Can you work these out from the model? Positions are in its coordinate system, mm. A direction names the side the tool comes from. Give positions to 0.01 mm unless a question says otherwise; leave off trailing zeros. Write each loop counter-clockwise with the first axis right and the second up, starting at its lowest first coordinate (ties: lowest second). Pieces come first, ordered by that corner, then holes. Notation, with made-up numbers: M 11,5.25 L 34,5.25 A17 ccw 34,36.25 Z; hole C -7,6.5 d10. An arc over 180 degrees is marked long. Write each question's results on one line, items separated by ' | '.
from build123d import *

# Parameters (mm, degrees)
SKETCH3_R           = 1
BOSS_EXTRUDE2_DEPTH = 3
BOSS_EXTRUDE5_DEPTH = 3


with BuildPart() as part:
    # Sketch3 → Boss-Extrude2 (new body)
    with BuildSketch(Plane.XY):
        with BuildLine():
            Line((-69.81, 20.47), (-34.625063383, 20.47))
            ThreePointArc((-34.625063383, 20.47), (-32.391172348, 20.03863815), (-30.478486436, 18.806576947))
            Line((-30.478486436, 18.806576947), (-26.141909489, 14.66))
            Line((-26.141909489, 14.66), (-1.5, 14.66))
            ThreePointArc((-1.5, 14.66), (2.742640687, 12.902640687), (4.5, 8.66))
            Line((4.5, 8.66), (4.5, 1.5))
            ThreePointArc((4.5, 1.5), (2.742640687, -2.742640687), (-1.5, -4.5))
            Line((-1.5, -4.5), (-26.141909489, -4.5))
            Line((-26.141909489, -4.5), (-30.478486436, -8.646576947))
            ThreePointArc((-30.478486436, -8.646576947), (-32.391172348, -9.87863815), (-34.625063383, -10.31))
            Line((-34.625063383, -10.31), (-69.81, -10.31))
            ThreePointArc((-69.81, -10.31), (-74.052640687, -8.552640687), (-75.81, -4.31))
            Line((-75.81, -4.31), (-75.81, 14.47))
            ThreePointArc((-75.81, 14.47), (-74.052640687, 18.712640687), (-69.81, 20.47))
        make_face()
        with Locations((-72.81, 17.47)):
            Circle(SKETCH3_R, mode=Mode.SUBTRACT)
        with Locations((-72.81, -7.31)):
            Circle(SKETCH3_R, mode=Mode.SUBTRACT)
        with Locations((1.5, -1.5)):
            Circle(SKETCH3_R, mode=Mode.SUBTRACT)
        with Locations((1.5, 11.66)):
            Circle(SKETCH3_R, mode=Mode.SUBTRACT)
        with BuildLine():
            Line((-69.81, 17.47), (-34.625063383, 17.47))
            ThreePointArc((-34.625063383, 17.47), (-33.508117866, 17.254319075), (-32.55177491, 16.638288474))
            Line((-32.55177491, 16.638288474), (-28.215197962, 12.491711526))
            ThreePointArc((-28.215197962, 12.491711526), (-27.258855006, 11.875680925), (-26.141909489, 11.66))
            Line((-26.141909489, 11.66), (-1.5, 11.66))
            ThreePointArc((-1.5, 11.66), (0.621320344, 10.781320344), (1.5, 8.66))
            Line((1.5, 8.66), (1.5, 1.5))
            ThreePointArc((1.5, 1.5), (0.621320344, -0.621320344), (-1.5, -1.5))
            Line((-1.5, -1.5), (-26.141909489, -1.5))
            ThreePointArc((-26.141909489, -1.5), (-27.258855006, -1.715680925), (-28.215197962, -2.331711526))
            Line((-28.215197962, -2.331711526), (-32.55177491, -6.478288474))
            ThreePointArc((-32.55177491, -6.478288474), (-33.508117866, -7.094319075), (-34.625063383, -7.31))
            Line((-34.625063383, -7.31), (-69.81, -7.31))
            ThreePointArc((-69.81, -7.31), (-71.931320344, -6.431320344), (-72.81, -4.31))
            Line((-72.81, -4.31), (-72.81, 14.47))
            ThreePointArc((-72.81, 14.47), (-71.931320344, 16.591320344), (-69.81, 17.47))
        make_face(mode=Mode.SUBTRACT)
    extrude(amount=BOSS_EXTRUDE2_DEPTH)

    # Sketch8 → Boss-Extrude5 (add)
    with BuildSketch(Plane.XY.offset(3)):
        with BuildLine():
            Line((-72.81, 14.47), (-72.81, -4.31))
            ThreePointArc((-72.81, -4.31), (-71.931320344, -6.431320344), (-69.81, -7.31))
            Line((-69.81, -7.31), (-34.625063383, -7.31))
            ThreePointArc((-34.625063383, -7.31), (-33.508117866, -7.094319075), (-32.55177491, -6.478288474))
            Line((-32.55177491, -6.478288474), (-28.215197962, -2.331711526))
            ThreePointArc((-28.215197962, -2.331711526), (-27.258855006, -1.715680925), (-26.141909489, -1.5))
            Line((-26.141909489, -1.5), (-1.5, -1.5))
            ThreePointArc((-1.5, -1.5), (0.621320344, -0.621320344), (1.5, 1.5))
            Line((1.5, 1.5), (1.5, 8.66))
            ThreePointArc((1.5, 8.66), (0.621320344, 10.781320344), (-1.5, 11.66))
            Line((-1.5, 11.66), (-26.141909489, 11.66))
            ThreePointArc((-26.141909489, 11.66), (-27.258855006, 11.875680925), (-28.215197962, 12.491711526))
            Line((-28.215197962, 12.491711526), (-32.55177491, 16.638288474))
            ThreePointArc((-32.55177491, 16.638288474), (-33.508117866, 17.254319075), (-34.625063383, 17.47))
            Line((-34.625063383, 17.47), (-69.81, 17.47))
            ThreePointArc((-69.81, 17.47), (-71.931320344, 16.591320344), (-72.81, 14.47))
        make_face()
    extrude(amount=-BOSS_EXTRUDE5_DEPTH)


solid = part.part
Item 1: I'm going to push flat-ended pins straight in: pin 1 (1.6 mm diameter, centred on x = 1.5, y = 11.66, fed in from -Z); pin 2 (1.5 mm diameter, centred on x = -15, z = 1.5, fed in from -Y); pin 3 (0.9 mm diameter, centred on x = -8, z = 1, fed in from +Y). Where does each tip first touch, or does it pass through?
Geometry says:
pin 1: passes through | pin 2: stops at y = -4.5 | pin 3: stops at y = 14.66
Item 2: I want a section at D-D, the plane y = 17.47. Please give me the cut outline in (x, z), and give its area (3 significant figures).
Geometry says:
outline: M -75.01,0 L -73.81,0 L -73.81,3 L -75.01,3 Z; M -71.81,0 L -29.08,0 L -29.08,3 L -71.81,3 Z | area: 132 mm2
Item 3: If I drill on line 1 (Y direction, x = -72.81, z = 1.2); line 2 (Y direction, x = 1.5, z = 1.6); line 3 (Y direction, x = -22, z = 0.5), over which ranges is the centre line in solid material (lowest first)? Write a range as from..to.
Geometry says:
line 1: y = -9.51..-8.31, -6.31..16.47, 18.47..19.67 | line 2: y = -3.7..-2.5, -0.5..10.66, 12.66..13.86 | line 3: y = -4.5..14.66
Item 4: I want a section at A-A, the plane z = 2.35. Please give me the cut outline in (x, y).
Geometry says:
outline: M -75.81,-4.31 A6 ccw -69.81,-10.31 L -34.63,-10.31 A6 ccw -30.48,-8.65 L -26.14,-4.5 L -1.5,-4.5 A6 ccw 4.5,1.5 L 4.5,8.66 A6 ccw -1.5,14.66 L -26.14,14.66 L -30.48,18.81 A6 ccw -34.63,20.47 L -69.81,20.47 A6 ccw -75.81,14.47 Z; hole C -72.81,-7.31 d2; hole C -72.81,17.47 d2; hole C 1.5,-1.5 d2; hole C 1.5,11.66 d2
Item 5: I want a section at B-B, the plane y = 11.66. Please give me the cut outline in (x, z).
Geometry says:
outline: M -75.81,0 L 0.5,0 L 0.5,3 L -75.81,3 Z; M 2.5,0 L 3.7,0 L 3.7,3 L 2.5,3 Z
Item 6: For faces 4 (the face through (-14, -4.5, 1)), 5 (the face through (-14, 14.66, 1)), 6 (the face through (1.283, -2.476, 1.479)), which set-ups out of +Z, -Z, +X, -X, +Y, -Y let a thin tool reach every point of the face, with its end or its side?
Geometry says:
face 4: +Z, -Z, +X, -Y | face 5: +Z, -Z, +X, +Y | face 6: +Z, -Z
Item 7: I want a section at C-C, the plane x = -72.81. Please give me the cut outline in (y, z), and give its area (3 significant figures).
Geometry says:
outline: M -9.51,0 L -8.31,0 L -8.31,3 L -9.51,3 Z; M -6.31,0 L 16.47,0 L 16.47,3 L -6.31,3 Z; M 18.47,0 L 19.67,0 L 19.67,3 L 18.47,3 Z | area: 75.5 mm2
Item 8: Thinking about a two-plate mould opening in Y: for faces 1 (the face through (-28.34, 16.76, 1.48)), 2 (the face through (2.789, -2.696, 1.479)), 3 (the face through (-73.6, 16.86, 1.48)), which applies, +Y half, -Y half, draft (parallel to the pull), parting line (faces both ways), or undercut?
Geometry says:
face 1: +Y half | face 2: -Y half | face 3: undercut
